Work out the finished part from the listing and answer in its coordinate system (mm). Coordinates: 2 decimals unless noted, no trailing zeros. Loops run counter-clockwise (first coordinate to the right, second up) from the corner with the lowest first, then second, coordinate; pieces in that order, holes last. Notation, with made-up numbers: (17.25, 76.25) -> (64.25, 76.25) arc R27 cw to (64.25, 101.25) -> close; hole circle Ø9 at (61, 3). An arc over 180 degrees is marked (long way). Answer as CSV lines item,"result".
```python
from build123d import *

# Parameters (mm, degrees)
F0_R     = 3.5687
F1_DEPTH = 1.5875


with BuildPart() as f1:
    # F0 (on Front) → F1 (new body, symmetric)
    with BuildSketch(Plane.XZ):
        with BuildLine():
            Line((-10.8839, 14.0208), (-8.0722359001, -1.4655733392))
            ThreePointArc((-8.0722359001, -1.4655733392), (0, -8.2042), (8.0722359001, -1.4655733392))
            Line((8.0722359001, -1.4655733392), (10.8839, 14.0208))
            Line((10.8839, 14.0208), (-10.8839, 14.0208))
        make_face()
        Circle(F0_R, mode=Mode.SUBTRACT)
    extrude(amount=F1_DEPTH, both=True)


solid = f1.part
```
(1) A cutting plane is placed at C-C, the plane y = 0.1. Write down the section's boundary in (x, z).
Computed values:
outline,"(-10.88, 14.02) -> (-8.07, -1.47) arc R8.2 ccw to (8.07, -1.47) -> (10.88, 14.02) -> close; hole circle Ø7.14 at (0, 0)"
(2) A cutting plane is placed at B-B, the plane z = 0. Write down the section's boundary in (x, y), and give its area (3 significant figures).
Computed values:
outline,"(-8.34, -1.59) -> (-3.57, -1.59) -> (-3.57, 1.59) -> (-8.34, 1.59) -> close; (3.57, -1.59) -> (8.34, -1.59) -> (8.34, 1.59) -> (3.57, 1.59) -> close"
area,"30.3 mm2"
(3) A cutting plane is placed at D-D, the plane x = -7. Write down the section's boundary in (y, z), and give its area (3 significant figures).
Computed values:
outline,"(-1.59, -4.28) -> (1.59, -4.28) -> (1.59, 14.02) -> (-1.59, 14.02) -> close"
area,"58.1 mm2"
(4) Flat-ended cylindrical pins translate along their axes: pin 1 Ø1 at (x, z) = (2.5, 0.5) entering from +Y; pin 2 Ø9.5 at (x, z) = (0, 0) entering from +Y; pin 3 Ø1 at (x, y) = (1, 1) entering from -Z. Find the tip coordinate at first contact, or state that the pin passes through.
Computed values:
pin 1,"through"
pin 2,"y = 1.59"
pin 3,"z = -8.19"
(5) A cutting plane is placed at A-A, the plane x = 0. Write down the section's boundary in (y, z).
Computed values:
outline,"(-1.59, -8.2) -> (1.59, -8.2) -> (1.59, -3.57) -> (-1.59, -3.57) -> close; (-1.59, 3.57) -> (1.59, 3.57) -> (1.59, 14.02) -> (-1.59, 14.02) -> close"
(6) For a pull along Z with two mould halves and no side action, classify faces 1 (the face through (9.46, -0.02, 6.17)), 2 (the face through (-3.565, 0.022, 0.157)), 3 (the face through (0, 0, 14.021)) as pulls with the +Z half, pulls with the -Z half, needs draft (parallel to the pull), parting line crosses it, or undercut.
Computed values:
face 1,"pulls with the -Z half"
face 2,"undercut"
face 3,"pulls with the +Z half"
(7) Consider line 1 along Z through (x, y) = (0, 0.65); line 2 along X through (y, z) = (0.5, -0.5); line 3 along X through (y, z) = (1.2, 2.5). Determine where each line is inside the solid, lowest interval first.
Computed values:
line 1,"-8.2 to -3.57, 3.57 to 14.02"
line 2,"-8.25 to -3.53, 3.53 to 8.25"
line 3,"-8.79 to -2.55, 2.55 to 8.79"
